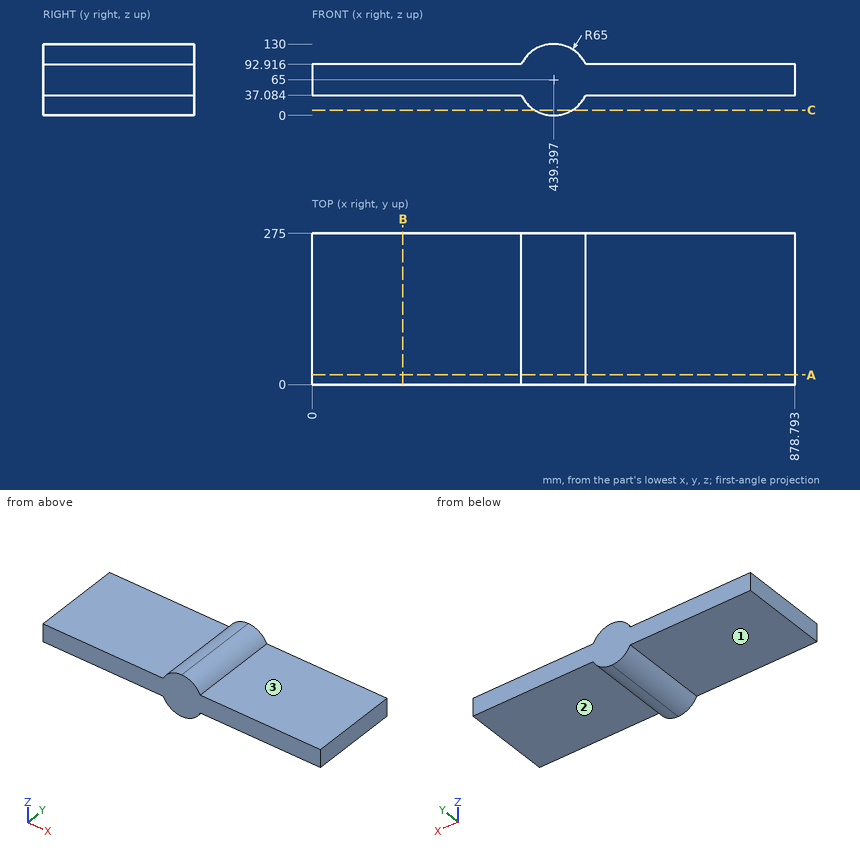
Geometry: see drawing. Coordinates: mm, zero at the bounding-box minimum. A direction names the side the tool comes from. Give positions to 0.01 mm unless a question says otherwise; leave off trailing zeros. Order: outer loops, then holes, each group sorted by start corner. A loop starts at its lowest first (then second) coordinate and runs counter-clockwise, first axis right, second up. Notation, with made-up numbers: (84, -1.5) - (115, -1.5) arc R22 ccw to (115, 15.5) - close; hole circle Ø11 at (14, 72). An arc over 180 degrees is marked (long way). Use a Markdown table: item, result.
(1) Pin query (flat end, axial travel): pin 1 (6 mm diameter, centred on x = 705.5, y = 221.5, fed in from +Z); pin 2 (3 mm diameter, centred on x = 594.5, y = 44, fed in from -Z). Return the tip coordinate at first contact, or that it passes through.
Computed values:
| item | result |
|---|---|
| pin 1 | stops at z = 92.92 |
| pin 2 | stops at z = 37.08 |
(2) Section query B-B (x = 165). Output: boundary loops of the cut face in (y, z).
Computed values:
| item | result |
|---|---|
| outline | (0, 37.08) - (275, 37.08) - (275, 92.92) - (0, 92.92) - close |
(3) Access query for the marked faces 1, 2 and 3. Directions: +Z, -Z, +X, -X, +Y, -Y. A direction counts if a zero-diameter tool reaches every point of the face in a straight line with its end or side. Return the directions, or none.
Computed values:
| item | result |
|---|---|
| face 1 | -Z, -X, +Y, -Y |
| face 2 | -Z, +X, +Y, -Y |
| face 3 | +Z, +X, +Y, -Y |
(4) Line query: line 1 (Z direction, x = 272, y = 176); line 2 (X direction, y = 240.5, z = 33) (1 decimal); line 3 (X direction, y = 68, z = 104) (1 decimal). Output: solid intervals per line, ascending. Write a range as from..to.
Computed values:
| item | result |
|---|---|
| line 1 | z = 37.08..92.92 |
| line 2 | x = 382.8..496 |
| line 3 | x = 387.4..491.4 |
(5) Section query C-C (z = 9.5). Output: boundary loops of the cut face in (x, y).
Computed values:
| item | result |
|---|---|
| outline | (405.56, 0) - (473.23, 0) - (473.23, 275) - (405.56, 275) - close |
(6) Section query A-A (y = 17.5). Output: boundary loops of the cut face in (x, z).
Computed values:
| item | result |
|---|---|
| outline | (0, 37.08) - (380.7, 37.08) arc R65 ccw to (439.4, 0) arc R65 ccw to (498.1, 37.08) - (878.79, 37.08) - (878.79, 92.92) - (498.1, 92.92) arc R65 ccw to (439.4, 130) arc R65 ccw to (380.7, 92.92) - (0, 92.92) - close |
